Model file for the job. Use its own axes, mm. Coordinates: 2 decimals unless noted, no trailing zeros. Order: outer loops, then holes, each group sorted by start corner. A loop starts at its lowest first (then second) coordinate and runs counter-clockwise, first axis right, second up.
from build123d import *

# Parameters (mm, degrees)
MAIN_EXTRUDE_DEPTH      = 2
SCREWHOLES_DEPTH        = 142.046534874
SCREWHOLES_DEPTH_BACK   = 142.046534874
SKETCH2_R               = 1
CUT_EXTRUDE2_DEPTH      = 142.046534874
CUT_EXTRUDE2_DEPTH_BACK = 142.046534874
SKETCH3_W               = 56
SKETCH3_H               = 83.75


with BuildPart() as part:
    # Sketch1 → Main extrude (new body)
    with BuildSketch(Plane.XY):
        with BuildLine():
            Line((-50, -51.75), (-50, -47))
            ThreePointArc((-50, -47), (-47.656854249, -41.343145751), (-42, -39))
            Line((-42, -39), (51, -39))
            ThreePointArc((51, -39), (56.656854249, -36.656854249), (59, -31))
            Line((59, -31), (59, 31.5))
            ThreePointArc((59, 31.5), (56.656854249, 37.156854249), (51, 39.5))
            Line((51, 39.5), (-119.75, 39.5))
            ThreePointArc((-119.75, 39.5), (-125.406854249, 37.156854249), (-127.75, 31.5))
            Line((-127.75, 31.5), (-127.75, -51.75))
            ThreePointArc((-127.75, -51.75), (-125.406854249, -57.406854249), (-119.75, -59.75))
            Line((-119.75, -59.75), (-58, -59.75))
            ThreePointArc((-58, -59.75), (-52.343145751, -57.406854249), (-50, -51.75))
        make_face()
    extrude(amount=MAIN_EXTRUDE_DEPTH)

    # Sketch2 → Screwholes (cut, two sides: drawn at the far end of the back side and taken through both)
    with BuildSketch(Plane.XY.offset(2).offset(-SCREWHOLES_DEPTH_BACK)):
        with Locations((-119.75, 31.5)):
            Circle(SKETCH2_R)
        with Locations((-119.75, -51.75)):
            Circle(SKETCH2_R)
    extrude(amount=SCREWHOLES_DEPTH + SCREWHOLES_DEPTH_BACK, mode=Mode.SUBTRACT)

    # Sketch3 → Cut-Extrude2 (cut, two sides: drawn at the far end of the back side and taken through both)
    with BuildSketch(Plane.XY.offset(2).offset(-CUT_EXTRUDE2_DEPTH_BACK)):
        with Locations((-85.25, -10.375)):
            Rectangle(SKETCH3_W, SKETCH3_H)
        with BuildLine():
            Line((-46, 27.5), (46, 27.5))
            ThreePointArc((46, 27.5), (48.121320344, 26.621320344), (49, 24.5))
            Line((49, 24.5), (49, -30))
            ThreePointArc((49, -30), (48.121320344, -32.121320344), (46, -33))
            Line((46, -33), (-46, -33))
            ThreePointArc((-46, -33), (-48.121320344, -32.121320344), (-49, -30))
            Line((-49, -30), (-49, 24.5))
            ThreePointArc((-49, 24.5), (-48.121320344, 26.621320344), (-46, 27.5))
        make_face()
    extrude(amount=CUT_EXTRUDE2_DEPTH + CUT_EXTRUDE2_DEPTH_BACK, mode=Mode.SUBTRACT)


solid = part.part
Q1. Cut at C-C, the plane y = 6. List the corners of the cut face in (x, z).
Established:
outline: (-127.75, 0) - (-113.25, 0) - (-113.25, 2) - (-127.75, 2) - close; (-57.25, 0) - (-49, 0) - (-49, 2) - (-57.25, 2) - close; (49, 0) - (59, 0) - (59, 2) - (49, 2) - close
Q2. Cut at A-A, the plane x = -83. List the corners of the cut face in (y, z).
Established:
outline: (-59.75, 0) - (-52.25, 0) - (-52.25, 2) - (-59.75, 2) - close; (31.5, 0) - (39.5, 0) - (39.5, 2) - (31.5, 2) - close
Q3. Probe line 1 (X direction, y = -10.5, z = 0.7); line 2 (Y direction, x = -119.75, z = 0.4); line 3 (X direction, y = -51.75, z = 1.1). List the from-to ranges inside material, lowest first.
Established:
line 1: x = -127.75 to -113.25, -57.25 to -49, 49 to 59
line 2: y = -59.75 to -52.75, -50.75 to 30.5, 32.5 to 39.5
line 3: x = -127.75 to -120.75, -118.75 to -113.25, -57.25 to -50
Q4. Drop flat-ended pins along their axis: P1, Ø1, axis at x = -12.5, z = 0.5, coming from the -Y side; P2, Ø12, axis at x = -66.5, y = -36.5, coming from the -Z side; P3, Ø5, axis at x = -47.5, y = 18.5, coming from the -Z side. Give the stop position or say it passes through.
Established:
P1: stops at y = -39
P2: passes through
P3: stops at z = 0
Q5. Cut at B-B, the plane z = 1.25. List the corners of the cut face in (x, y).
Established:
outline: (-127.75, -51.75) arc R8 ccw to (-119.75, -59.75) - (-58, -59.75) arc R8 ccw to (-50, -51.75) - (-50, -47) arc R8 cw to (-42, -39) - (51, -39) arc R8 ccw to (59, -31) - (59, 31.5) arc R8 ccw to (51, 39.5) - (-119.75, 39.5) arc R8 ccw to (-127.75, 31.5) - close; hole circle Ø2 at (-119.75, -51.75); hole circle Ø2 at (-119.75, 31.5); hole (-113.25, -52.25) - (-57.25, -52.25) - (-57.25, 31.5) - (-113.25, 31.5) - close; hole (-49, -30) arc R3 ccw to (-46, -33) - (46, -33) arc R3 ccw to (49, -30) - (49, 24.5) arc R3 ccw to (46, 27.5) - (-46, 27.5) arc R3 ccw to (-49, 24.5) - close
Q6. Cut at D-D, the plane x = -32. List the corners of the cut face in (y, z), plus the area to 3 significant figures.
Established:
outline: (-39, 0) - (-33, 0) - (-33, 2) - (-39, 2) - close; (27.5, 0) - (39.5, 0) - (39.5, 2) - (27.5, 2) - close
area: 36.0 mm2
